Geometry: final body of the model. Coordinates: model frame, mm. Face numbers are marked on the shaded views. A direction names the side the tool comes from. Give positions to 0.01 mm unless a question says otherwise; leave off trailing zeros. Write each loop counter-clockwise with the first axis right and the second up, starting at its lowest first coordinate (ties: lowest second). Pieces come first, ordered by that corner, then holes. Notation, with made-up numbers: (15, -38) - (27, -38) arc R18 ccw to (27, -32) - close; hole circle Ø1 at (33.25, -1.75). An arc over 180 degrees is marked (long way). Return JSON: item names as keys, results as strings.
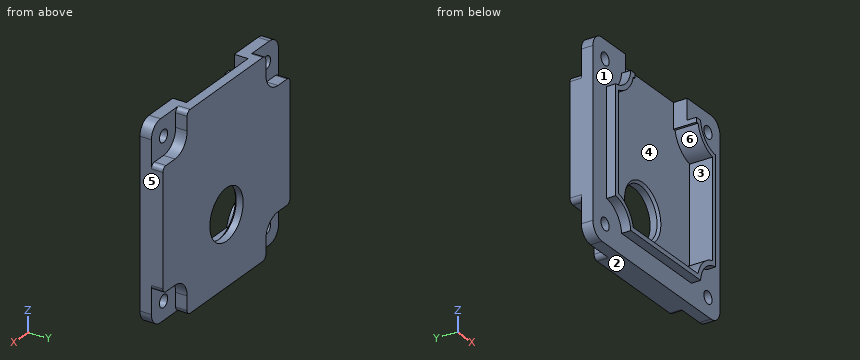
from build123d import *

# Parameters (mm, degrees)
SKETCH2_W           = 42
SKETCH2_H           = 42
SKETCH2_R           = 5.5
BOSS_EXTRUDE1_DEPTH = 2
SKETCH4_W           = 42
SKETCH4_H           = 42
BOSS_EXTRUDE2_DEPTH = 3
BOSS_EXTRUDE3_DEPTH = 3
BOSS_EXTRUDE5_DEPTH = 5
CUT_EXTRUDE1_DEPTH  = 2.5
SKETCH9_R           = 1.35
CUT_EXTRUDE2_DEPTH  = 8
FILLET1_R           = 3
FILLET2_R           = 1
CHAMFER1_SIZE       = 0.5
SKETCH10_W          = 20.32
SKETCH10_H          = 5
CUT_EXTRUDE3_DEPTH  = 5.5


with BuildPart() as part:
    # Sketch2 → Boss-Extrude1 (new body)
    with BuildSketch(Plane(origin=(0, 0, 0), x_dir=(1, 0, 0), z_dir=(0, 1, 0))):
        Rectangle(SKETCH2_W, SKETCH2_H)
        with Locations((0, 6)):
            Circle(SKETCH2_R, mode=Mode.SUBTRACT)
    extrude(amount=-BOSS_EXTRUDE1_DEPTH)

    # Sketch4 → Boss-Extrude2 (add)
    with BuildSketch(Plane.XZ.offset(2)):
        Rectangle(SKETCH4_W, SKETCH4_H)
        with BuildLine():
            Line((-17, 11.522774425), (-17, -11.522774425))
            ThreePointArc((-17, -11.522774425), (-16.869274473, -11.859874356), (-16.545454545, -12.020704023))
            ThreePointArc((-16.545454545, -12.020704023), (-13.464466094, -13.464466094), (-12.020704023, -16.545454545))
            ThreePointArc((-12.020704023, -16.545454545), (-11.859874356, -16.869274473), (-11.522774425, -17))
            Line((-11.522774425, -17), (11.522774425, -17))
            ThreePointArc((11.522774425, -17), (11.859874356, -16.869274473), (12.020704023, -16.545454545))
            ThreePointArc((12.020704023, -16.545454545), (13.464466094, -13.464466094), (16.545454545, -12.020704023))
            ThreePointArc((16.545454545, -12.020704023), (16.869274473, -11.859874356), (17, -11.522774425))
            Line((17, -11.522774425), (17, 11.522774425))
            ThreePointArc((17, 11.522774425), (16.869274473, 11.859874356), (16.545454545, 12.020704023))
            ThreePointArc((16.545454545, 12.020704023), (13.464466094, 13.464466094), (12.020704023, 16.545454545))
            ThreePointArc((12.020704023, 16.545454545), (11.859874356, 16.869274473), (11.522774425, 17))
            Line((11.522774425, 17), (-11.522774425, 17))
            ThreePointArc((-11.522774425, 17), (-11.859874356, 16.869274473), (-12.020704023, 16.545454545))
            ThreePointArc((-12.020704023, 16.545454545), (-13.464466094, 13.464466094), (-16.545454545, 12.020704023))
            ThreePointArc((-16.545454545, 12.020704023), (-16.869274473, 11.859874356), (-17, 11.522774425))
        make_face(mode=Mode.SUBTRACT)
    extrude(amount=BOSS_EXTRUDE2_DEPTH)

    # Sketch6 → Boss-Extrude3 (add)
    with BuildSketch(Plane.XZ.offset(2)):
        with BuildLine():
            Line((-17, 11.522774425), (-17, -11.522774425))
            ThreePointArc((-17, -11.522774425), (-16.869274473, -11.859874356), (-16.545454545, -12.020704023))
            ThreePointArc((-16.545454545, -12.020704023), (-13.464466094, -13.464466094), (-12.020704023, -16.545454545))
            ThreePointArc((-12.020704023, -16.545454545), (-11.859874356, -16.869274473), (-11.522774425, -17))
            Line((-11.522774425, -17), (11.522774425, -17))
            ThreePointArc((11.522774425, -17), (11.859874356, -16.869274473), (12.020704023, -16.545454545))
            ThreePointArc((12.020704023, -16.545454545), (13.464466094, -13.464466094), (16.545454545, -12.020704023))
            ThreePointArc((16.545454545, -12.020704023), (16.869274473, -11.859874356), (17, -11.522774425))
            Line((17, -11.522774425), (17, 11.522774425))
            ThreePointArc((17, 11.522774425), (16.869274473, 11.859874356), (16.545454545, 12.020704023))
            ThreePointArc((16.545454545, 12.020704023), (13.464466094, 13.464466094), (12.020704023, 16.545454545))
            ThreePointArc((12.020704023, 16.545454545), (11.859874356, 16.869274473), (11.522774425, 17))
            Line((11.522774425, 17), (-11.522774425, 17))
            ThreePointArc((-11.522774425, 17), (-11.859874356, 16.869274473), (-12.020704023, 16.545454545))
            ThreePointArc((-12.020704023, 16.545454545), (-13.464466094, 13.464466094), (-16.545454545, 12.020704023))
            ThreePointArc((-16.545454545, 12.020704023), (-16.869274473, 11.859874356), (-17, 11.522774425))
        make_face()
        with BuildLine():
            Line((-16.5, 11.522774425), (-16.5, -11.522774425))
            ThreePointArc((-16.5, -11.522774425), (-13.110912703, -13.110912703), (-11.522774425, -16.5))
            Line((-11.522774425, -16.5), (11.522774425, -16.5))
            ThreePointArc((11.522774425, -16.5), (13.110912703, -13.110912703), (16.5, -11.522774425))
            Line((16.5, -11.522774425), (16.5, 11.522774425))
            ThreePointArc((16.5, 11.522774425), (13.110912703, 13.110912703), (11.522774425, 16.5))
            Line((11.522774425, 16.5), (-11.522774425, 16.5))
            ThreePointArc((-11.522774425, 16.5), (-13.110912703, 13.110912703), (-16.5, 11.522774425))
        make_face(mode=Mode.SUBTRACT)
    extrude(amount=BOSS_EXTRUDE3_DEPTH)

    # Sketch7 → Boss-Extrude5 (add)
    with BuildSketch(Plane.XZ.offset(2)):
        with BuildLine():
            Line((11.522774425, 16.5), (-11.522774425, 16.5))
            ThreePointArc((-11.522774425, 16.5), (-13.110912703, 13.110912703), (-16.5, 11.522774425))
            Line((-16.5, 11.522774425), (-16.5, -11.522774425))
            ThreePointArc((-16.5, -11.522774425), (-13.110912703, -13.110912703), (-11.522774425, -16.5))
            Line((-11.522774425, -16.5), (11.522774425, -16.5))
            ThreePointArc((11.522774425, -16.5), (13.110912703, -13.110912703), (16.5, -11.522774425))
            Line((16.5, -11.522774425), (16.5, 11.522774425))
            ThreePointArc((16.5, 11.522774425), (13.110912703, 13.110912703), (11.522774425, 16.5))
        make_face()
        with BuildLine():
            Line((10.67544468, 15.5), (-10.67544468, 15.5))
            ThreePointArc((-10.67544468, 15.5), (-12.403805922, 12.403805922), (-15.5, 10.67544468))
            Line((-15.5, 10.67544468), (-15.5, -10.67544468))
            ThreePointArc((-15.5, -10.67544468), (-12.403805922, -12.403805922), (-10.67544468, -15.5))
            Line((-10.67544468, -15.5), (10.67544468, -15.5))
            ThreePointArc((10.67544468, -15.5), (12.403805922, -12.403805922), (15.5, -10.67544468))
            Line((15.5, -10.67544468), (15.5, 10.67544468))
            ThreePointArc((15.5, 10.67544468), (12.403805922, 12.403805922), (10.67544468, 15.5))
        make_face(mode=Mode.SUBTRACT)
    extrude(amount=BOSS_EXTRUDE5_DEPTH)

    # Sketch8 → Cut-Extrude1 (cut)
    with BuildSketch(Plane(origin=(0, 0, 0), x_dir=(1, 0, 0), z_dir=(0, 1, 0))):
        with BuildLine():
            Line((-17, 13), (-21, 13))
            Line((-21, 13), (-21, 21))
            Line((-21, 21), (-13, 21))
            Line((-13, 21), (-13, 17))
            ThreePointArc((-13, 17), (-14.171572875, 14.171572875), (-17, 13))
        make_face()
        with BuildLine():
            Line((13, 17), (13, 21))
            Line((13, 21), (21, 21))
            Line((21, 21), (21, 13))
            Line((21, 13), (17, 13))
            ThreePointArc((17, 13), (14.171572875, 14.171572875), (13, 17))
        make_face()
        with BuildLine():
            Line((-21, -17), (-21, -21))
            Line((-21, -21), (-17, -21))
            Line((-17, -21), (-13, -21))
            Line((-13, -21), (-13, -17))
            ThreePointArc((-13, -17), (-14.171572875, -14.171572875), (-17, -13))
            Line((-17, -13), (-21, -13))
            Line((-21, -13), (-21, -17))
        make_face()
        with BuildLine():
            Line((17, -13), (21, -13))
            Line((21, -13), (21, -21))
            Line((21, -21), (17, -21))
            Line((17, -21), (13, -21))
            Line((13, -21), (13, -17))
            ThreePointArc((13, -17), (14.171572875, -14.171572875), (17, -13))
        make_face()
    extrude(amount=-CUT_EXTRUDE1_DEPTH, mode=Mode.SUBTRACT)

    # Sketch9 → Cut-Extrude2 (cut, through all)
    with BuildSketch(Plane(origin=(0, 0, 0), x_dir=(1, 0, 0), z_dir=(0, 1, 0))):
        with Locations((-17, 17)):
            Circle(SKETCH9_R)
        with Locations((17, 17)):
            Circle(SKETCH9_R)
        with Locations((-17, -17)):
            Circle(SKETCH9_R)
        with Locations((17, -17)):
            Circle(SKETCH9_R)
    extrude(amount=-CUT_EXTRUDE2_DEPTH, mode=Mode.SUBTRACT)

    # Fillet1
    fillet1_edges = [part.edges().sort_by_distance(p)[0] for p in [
        (21, -3.75, 21),
        (-21, -3.75, 21),
        (-21, -3.75, -21),
        (21, -3.75, -21),
    ]]
    fillet(fillet1_edges, radius=FILLET1_R)

    # Fillet2
    fillet2_edges = [part.edges().sort_by_distance(p)[0] for p in [
        (13, -1.25, -21),
        (21, -1.25, -13),
        (-21, -1.25, 13),
        (-13, -1.25, 21),
        (21, -1.25, 13),
        (13, -1.25, 21),
        (-21, -1.25, -13),
        (-13, -1.25, -21),
    ]]
    fillet(fillet2_edges, radius=FILLET2_R)

    # Chamfer1
    chamfer1_edges = [part.edges().sort_by_distance(p)[0] for p in [
        (-5.5, -2, -6),
    ]]
    chamfer(chamfer1_edges, length=CHAMFER1_SIZE)

    # Sketch10 → Cut-Extrude3 (cut)
    with BuildSketch(Plane.XY.offset(21)):
        with Locations((0, -4.5)):
            Rectangle(SKETCH10_W, SKETCH10_H)
    extrude(amount=-CUT_EXTRUDE3_DEPTH, mode=Mode.SUBTRACT)


solid = part.part
Q1. Section query A-A, the plane z = -6. Return the cut outline in (x, y).
Answer key:
{"outline": "(-21, -5) - (-16.5, -5) - (-16.5, -7) - (-15.5, -7) - (-15.5, -2) - (-6, -2) - (-5.5, -1.5) - (-5.5, 0) - (-21, 0) - close; (5.5, -1.5) - (6, -2) - (15.5, -2) - (15.5, -7) - (16.5, -7) - (16.5, -5) - (21, -5) - (21, 0) - (5.5, 0) - close"}
Q2. Section query D-D, the plane y = -0.5. Return the cut outline in (x, z).
Answer key:
{"outline": "(-21, -12) arc R1 ccw to (-20, -13) - (-17, -13) arc R4 cw to (-13, -17) - (-13, -20) arc R1 ccw to (-12, -21) - (12, -21) arc R1 ccw to (13, -20) - (13, -17) arc R4 cw to (17, -13) - (20, -13) arc R1 ccw to (21, -12) - (21, 12) arc R1 ccw to (20, 13) - (17, 13) arc R4 cw to (13, 17) - (13, 20) arc R1 ccw to (12, 21) - (-12, 21) arc R1 ccw to (-13, 20) - (-13, 17) arc R4 cw to (-17, 13) - (-20, 13) arc R1 ccw to (-21, 12) - close; hole circle Ø11 at (0, -6)"}
Q3. Section query B-B, the plane y = -3.5. Return the cut outline in (x, z).
Answer key:
{"outline": "(-21, -18) arc R3 ccw to (-18, -21) - (18, -21) arc R3 ccw to (21, -18) - (21, 18) arc R3 ccw to (18, 21) - (10.16, 21) - (10.16, 15.5) - (10.68, 15.5) arc R6.5 ccw to (15.5, 10.68) - (15.5, -10.68) arc R6.5 ccw to (10.68, -15.5) - (-10.68, -15.5) arc R6.5 ccw to (-15.5, -10.68) - (-15.5, 10.68) arc R6.5 ccw to (-10.68, 15.5) - (-10.16, 15.5) - (-10.16, 21) - (-18, 21) arc R3 ccw to (-21, 18) - close; hole circle Ø2.7 at (-17, -17); hole circle Ø2.7 at (-17, 17); hole circle Ø2.7 at (17, -17); hole circle Ø2.7 at (17, 17)"}
Q4. Mould query, pull axis Z, two halves, no side actions, for the marked faces 1, 2, 3 and 4. Classes: pulls with the +Z half, pulls with the -Z half, needs draft (parallel to the pull), parting line crosses it, or undercut.
Answer key:
{"face 1": "needs draft", "face 2": "pulls with the -Z half", "face 3": "undercut", "face 4": "undercut"}
Q5. Pin query (flat end, axial travel): P1, Ø3, axis at y = -0.5, z = 18, coming from the -X side; P2, Ø4.5, axis at x = 17, z = 17, coming from the +Y side; P3, Ø1.2, axis at x = -19, y = -1.5, coming from the +Z side. Return the tip coordinate at first contact, or that it passes through.
Answer key:
{"P1": "stops at x = -13.03", "P2": "stops at y = -2.5", "P3": "stops at z = 13"}
Q6. Material intervals for probe 1 along Z at (x, y) = (-17, -4.4); probe 2 along Z at (x, y) = (0, -0.35), sorted ascending. Write a range as [from, to].
Answer key:
{"probe 1": "z = [-21, -18.35], [-15.65, 15.65], [18.35, 21]", "probe 2": "z = [-21, -11.5], [-0.5, 21]"}
Q7. Section query C-C, the plane x = 0. Return the cut outline in (y, z).
Answer key:
{"outline": "(-7, -16.5) - (-5, -16.5) - (-5, -21) - (0, -21) - (0, -11.5) - (-1.5, -11.5) - (-2, -12) - (-2, -15.5) - (-7, -15.5) - close; (-2, 0) - (-1.5, -0.5) - (0, -0.5) - (0, 21) - (-2, 21) - close"}
Q8. Set-up query: the marked faces 5 and 6. Return all of +Z, -Z, +X, -X, +Y, -Y with unobstructed straight access to the full face (end or side cutting, diameter ignored); none if empty.
Answer key:
{"face 5": "+Z, -Z, +X, +Y, -Y", "face 6": "-Y"}
